Build history of the part. All positions in model axes, mm. A direction names the side the tool comes from. Give positions to 0.01 mm unless a question says otherwise; leave off trailing zeros. Write each loop counter-clockwise with the first axis right and the second up, starting at its lowest first coordinate (ties: lowest second). Pieces come first, ordered by that corner, then holes. Notation, with made-up numbers: (-30.75, -19) -> (17.25, -19) arc R20 cw to (17.25, -4) -> close; hole circle Ø10 at (4, 2.25). An arc over 180 degrees is marked (long way). One line per question, with ' | ' between items. Start each with the question number.
(1) Band-saw the part on D-D, the plane z = 2.5. Give the cut face in (x, y).
(2) Drill centre lines: probe 1 along Z at (x, y) = (0.5, 2.5); probe 2 along Z at (x, y) = (-3.5, -6.75); probe 3 along X at (y, z) = (-0.25, 6). Where is each one in solid material? Low to high. Write a range as from..to.
(3) Band-saw the part on C-C, the plane z = 8.5. Give the cut face in (x, y).
(4) Tool access for faces 1 (the flat face through (0, 0, 0)), 2 (the flat face through (5, -2, 3.5)): list every direction of +Z, -Z, +X, -X, +Y, -Y with a clear straight run to the whole face (end or side of a thin tool).
(5) Pin check, flat tips, straight feed: P1, Ø5, axis at x = -8, z = 2.5, coming from the +Y side; P2, Ø6, axis at x = -8.5, y = -5, coming from the +Z side; P3, Ø6.5, axis at x = -5, y = 4.5, coming from the +Z side. Stop position of each tip, or through.
from build123d import *

# Parameters (mm, degrees)
F0_R      = 12
F0_R_2    = 11
F0_R_3    = 5
F0_R_4    = 4.1
F0_R_5    = 3
F1_DEPTH  = 2
F2_DEPTH  = 3.5
F3_SIZE   = 0.99999
F4_DEPTH  = 4.5
F5_DEPTH  = 7.5
F6_DEPTH  = 10
F7_SIZE   = 1
F8_SIZE   = 0.5
F9_R      = 3
F9_R_2    = 2.5
F10_DEPTH = 2.5
F11_R     = 4.1
F11_R_2   = 3.6
F12_DEPTH = 3


# Not quite as in the source:
# - a fillet or chamfer is up to 0.001 mm smaller than in the source, because OpenCascade refuses the exact size


with BuildPart() as f1:
    # F0 (on Top) → F1 (new body)
    with BuildSketch(Plane.XY):
        Circle(F0_R)
        Circle(F0_R_2, mode=Mode.SUBTRACT)
        Circle(F0_R_2)
        Circle(F0_R_3, mode=Mode.SUBTRACT)
        Circle(F0_R_3)
        Circle(F0_R_4, mode=Mode.SUBTRACT)
        Circle(F0_R_4)
        Circle(F0_R_5, mode=Mode.SUBTRACT)
        Circle(F0_R_5)
    extrude(amount=F1_DEPTH)

    # F0 (on Top) → F2 (join)
    with BuildSketch(Plane.XY):
        Circle(F0_R_2)
        Circle(F0_R_3, mode=Mode.SUBTRACT)
        Circle(F0_R_3)
        Circle(F0_R_4, mode=Mode.SUBTRACT)
        Circle(F0_R_4)
        Circle(F0_R_5, mode=Mode.SUBTRACT)
        Circle(F0_R_5)
    extrude(amount=F2_DEPTH)

    # F3 (size 1 in the source; OpenCascade refuses exactly that, so slightly less here)
    f3_edges = [f1.edges().sort_by_distance(p)[0] for p in [
        (-11, 0, 2),
    ]]
    chamfer(f3_edges, length=F3_SIZE)

    # F0 (on Top) → F4 (join)
    with BuildSketch(Plane.XY):
        Circle(F0_R_3)
        Circle(F0_R_4, mode=Mode.SUBTRACT)
        Circle(F0_R_4)
        Circle(F0_R_5, mode=Mode.SUBTRACT)
        Circle(F0_R_5)
    extrude(amount=F4_DEPTH)

    # F0 (on Top) → F5 (join)
    with BuildSketch(Plane.XY):
        Circle(F0_R_4)
        Circle(F0_R_5, mode=Mode.SUBTRACT)
    extrude(amount=F5_DEPTH)

    # F0 (on Top) → F6 (join)
    with BuildSketch(Plane.XY):
        Circle(F0_R_5)
    extrude(amount=F6_DEPTH)

    # F7
    f7_edges = [f1.edges().sort_by_distance(p)[0] for p in [
        (-12, 0, 0),
    ]]
    chamfer(f7_edges, length=F7_SIZE)

    # F8
    f8_edges = [f1.edges().sort_by_distance(p)[0] for p in [
        (-11, 0, 3.5),
    ]]
    chamfer(f8_edges, length=F8_SIZE)

    # F9 (on face) → F10 (cut, through all)
    with BuildSketch(Plane.XY.offset(10)):
        Circle(F9_R)
        Circle(F9_R_2, mode=Mode.SUBTRACT)
    extrude(amount=-F10_DEPTH, mode=Mode.SUBTRACT)

    # F11 (on face) → F12 (cut, through all)
    with BuildSketch(Plane.XY.offset(7.5)):
        Circle(F11_R)
        Circle(F11_R_2, mode=Mode.SUBTRACT)
    extrude(amount=-F12_DEPTH, mode=Mode.SUBTRACT)


solid = f1.part
Results:
1) outline: circle Ø23 at (0, 0)
2) probe 1: z = 0..7.5 | probe 2: z = 0..3.5 | probe 3: x = -3.59..3.59
3) outline: circle Ø5 at (0, 0)
4) face 1: -Z, +X, -X, +Y, -Y | face 2: +Z
5) P1: stops at y = 10.64 | P2: stops at z = 3.5 | P3: stops at z = 7.5
